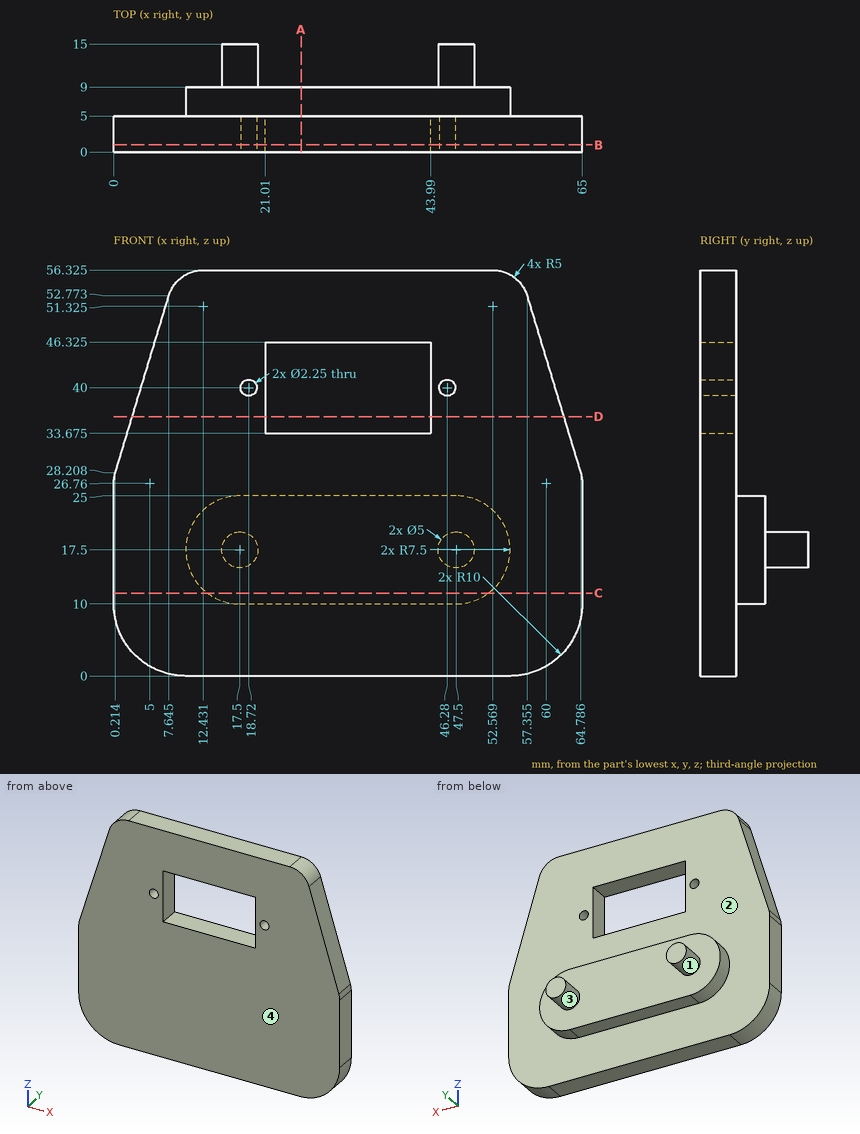
The drawing under review shows one solid part. Ordinate dimensions are in mm from its lowest x, y, z. A direction names the side the tool comes from. Round coordinates to 2 decimals unless told otherwise and drop trailing zeros. Loops run counter-clockwise (first coordinate to the right, second up) from the corner with the lowest first, then second, coordinate; pieces in that order, holes last. Notation, with made-up numbers: (8, 19.5) - (62, 19.5) arc R16 cw to (62, 48.5) - close; hole circle Ø11 at (-4, 8). An arc over 180 degrees is marked (long way). One line per question, with ' | ' between items.
Q1. Take a section at D-D (z = 36). Give the boundary of the cut face in (x, y), and give its area (3 significant figures).
Taken from the geometry:
outline: (2.57, 0) - (21.01, 0) - (21.01, 5) - (2.57, 5) - close; (43.99, 0) - (62.43, 0) - (62.43, 5) - (43.99, 5) - close | area: 184 mm²
Q2. Tool access review of the marked faces 3 and 4: name each direction out of +Z, -Z, +X, -X, +Y, -Y from which nothing blocks a thin tool from reaching the whole face with its end or side.
Taken from the geometry:
face 3: +Y | face 4: +Z, -Z, +X, -X, -Y
Q3. For pin 1 (5.5 mm diameter, centred on x = 32.5, y = 2.5, fed in from -Z); pin 2 (2.5 mm diameter, centred on x = 46.28, z = 40, fed in from +Y); pin 3 (1 mm diameter, centred on y = 9, z = 17.5, fed in from +X); pin 4 (5.5 mm diameter, centred on y = 3.5, z = 39, fed in from +X), all flat-tipped, find the tip position at first contact; note any pin that passes through.
Taken from the geometry:
pin 1: stops at z = 0 | pin 2: stops at y = 5 | pin 3: stops at x = 55 | pin 4: stops at x = 62.35
Q4. The part is to be moulded in two halves that separate along X. For the marked faces 1 and 2, say which applies: released by +X, released by -X, zero draft, split by the parting line, or undercut.
Taken from the geometry:
face 1: undercut | face 2: zero draft
Q5. Take a section at B-B (y = 1). State how many separate pieces and enclosed holes the cut face has, and give its area (3 significant figures).
Taken from the geometry:
separate pieces: 1 | enclosed holes: 3 | area: 3,060 mm²
Q6. For line 1 along Z through (x, y) = (30.5, 1.25) (1 decimal); line 2 along X through (y, z) = (3.65, 40) (1 decimal); line 3 along Y through (x, z) = (31.5, 25.5), list the stretches that pass through material, from the lowest coordinate up. Write a range as [from, to].
Taken from the geometry:
line 1: z = [0, 33.7], [46.3, 56.3] | line 2: x = [3.8, 17.6], [19.8, 21], [44, 45.2], [47.4, 61.2] | line 3: y = [0, 5]
Q7. Take a section at C-C (z = 11.5). Give the boundary of the cut face in (x, y), and give its area (3 significant figures).
Taken from the geometry:
outline: (0, 0) - (65, 0) - (65, 5) - (52, 5) - (52, 9) - (13, 9) - (13, 5) - (0, 5) - close | area: 481 mm²
Q8. Take a section at A-A (x = 26). Give the boundary of the cut face in (y, z) (1 decimal).
Taken from the geometry:
outline: (0, 0) - (5, 0) - (5, 10) - (9, 10) - (9, 25) - (5, 25) - (5, 33.7) - (0, 33.7) - close; (0, 46.3) - (5, 46.3) - (5, 56.3) - (0, 56.3) - close
